```python
from build123d import *

# Parameters (mm, degrees)
EXTRUDE_1_DEPTH     = 20
SKETCH_2_R          = 1.1
CUT_EXTRUDE_2_DEPTH = 27.248809497
CUT_EXTRUDE_3_REACH = 31.682
SKETCH_3_W          = 30
SKETCH_3_H          = 15.1
FILLET_1_R          = 3
SKETCH_6_W          = 30.918408881
SKETCH_6_H          = 20
SKETCH_6_W_2        = 27.918408881
SKETCH_6_H_2        = 17
EXTRUDE_2_DEPTH     = 2.5
FILLET_2_R          = 3.5


with BuildPart() as part:
    # 草图1 → 凸台-拉伸1 (new body)
    with BuildSketch(Plane(origin=(0, 0, 0), x_dir=(1, 0, 0), z_dir=(0, 1, 0))):
        Polygon((-15, -8), (15, -0.520159915), (15, 8), (-15, 8), align=None)
    extrude(amount=EXTRUDE_1_DEPTH)

    # 草图2 → 切除-拉伸2 (cut, through all)
    with BuildSketch(Plane(origin=(0, 20, 0), x_dir=(1, 0, 0), z_dir=(0, 1, 0))):
        with Locations(Location((-13, 2, 0), (0, 0, 270))):
            Circle(SKETCH_2_R)
        with Locations(Location((-8.332097868, 3.791839748, 0), (0, 0, 270))):
            Circle(SKETCH_2_R)
        with Locations(Location((-3.664195735, 5.583679495, 0), (0, 0, 270))):
            Circle(SKETCH_2_R)
    extrude(amount=-CUT_EXTRUDE_2_DEPTH, mode=Mode.SUBTRACT)

    # 切除-拉伸3: up to this plane
    cut_extrude_3_end = Plane(origin=(0.637110354, 0, 2.555310061), z_dir=(0.24192189559966876, 0, 0.9702957262759963))
    # 草图3 → 切除-拉伸3 (cut, up to the surface)
    with BuildSketch(Plane(origin=(0, 0, -8), x_dir=(-1, 0, 0), z_dir=(0, 0, -1)), mode=Mode.PRIVATE) as cut_extrude_3_sk1:
        with Locations((0, 10)):
            Rectangle(SKETCH_3_W, SKETCH_3_H)
    cut_extrude_3_tool1 = split(extrude(cut_extrude_3_sk1.sketch, amount=-CUT_EXTRUDE_3_REACH, mode=Mode.PRIVATE), bisect_by=cut_extrude_3_end, keep=Keep.BOTH, mode=Mode.PRIVATE)
    add(cut_extrude_3_tool1.solids().sort_by_distance((0, 10, -8))[0], mode=Mode.SUBTRACT)

    # 圆角1
    fillet_1_edges = [part.edges().sort_by_distance(p)[0] for p in [
        (-15, 1.225, -8),
        (-15, 18.775, -8),
    ]]
    fillet(fillet_1_edges, radius=FILLET_1_R)

    # 草图6 → 凸台-拉伸2 (add)
    with BuildSketch(Plane(origin=(0.999993198, 0, 4.010753651), x_dir=(0.9702957262759964, 0, -0.2419218955996687), z_dir=(0.2419218955996687, 0, 0.9702957262759964))):
        with Locations((-1.030606619, 10)):
            Rectangle(SKETCH_6_W, SKETCH_6_H)
        with Locations((-1.030606619, 10)):
            Rectangle(SKETCH_6_W_2, SKETCH_6_H_2, mode=Mode.SUBTRACT)
    extrude(amount=EXTRUDE_2_DEPTH)

    # 圆角2
    fillet_2_edges = [part.edges().sort_by_distance(p)[0] for p in [
        (15, 1.225, -8),
        (15, 18.775, -8),
    ]]
    fillet(fillet_2_edges, radius=FILLET_2_R)


solid = part.part
```
Work out the finished part from the listing and answer in its coordinate system (mm). A direction names the side the tool comes from. Round coordinates to 2 decimals unless told otherwise and drop trailing zeros. Write each loop counter-clockwise with the first axis right and the second up, starting at its lowest first coordinate (ties: lowest second). Pieces come first, ordered by that corner, then holes.
1) Consider probe 1 along Y at (x, z) = (-11, 9); probe 2 along Y at (x, z) = (-6, -2.75); probe 3 along X at (y, z) = (1.85, -2). Determine where each line is inside the solid, lowest interval first.
2) Which of the six approach directions +Z, -Z, +X, -X, +Y, -Y give full straight-line access (tool end or side, diameter ignored) to faces 4 (the face through (0, 17.55, -2)), 5 (the face through (-13.246, 9.881, 8.833)), 6 (the face through (-3.616, 18.792, -6.683)), 7 (the face through (0, 19, -8)), 8 (the face through (13.843, 9.881, 2.079))?
3) Determine the mould class of faces 1 (the face through (-8.753, 1.242, -2.776)), 2 (the face through (-14.7, 9.9, 9.2)), 3 (the face through (-1, 0, 0)) for opening direction Z: pulls with the +Z half, pulls with the -Z half, needs draft (parallel to the pull), parting line crosses it, or undercut.
4) A cutting plane is placed at C-C on y = 4.5. Determine the outline of the cut face in (x, z), and give its area (3 significant figures).
5) A cutting plane is placed at A-A on z = -2. Determine the outline of the cut face in (x, y), and give its area (3 significant figures).
6) Flat-ended cylindrical pins translate along their axes: P1, Ø1.8, axis at x = -3.66, z = -5.58, coming from the -Y side; P2, Ø12, axis at x = 4.5, y = 9, coming from the +Z side. Find the tip coordinate at first contact, or state that the pin passes through.
7) A cutting plane is placed at D-D on z = 1.25. Determine the outline of the cut face in (x, y).
8) A cutting plane is placed at B-B on x = -12.5. Determine the outline of the cut face in (y, z), and give its area (3 significant figures).
Entries:
1. probe 1: y = 0 to 1.5, 18.5 to 20
1. probe 2: y = 0 to 2.45, 17.55 to 20
1. probe 3: x = -15 to -14.1, -11.9 to 15
2. face 4: -Z, -X
2. face 5: +X
2. face 6: +Y, -Y
2. face 7: -Z, +X, -X, +Y, -Y
2. face 8: +Z
3. face 1: undercut
3. face 2: pulls with the +Z half
3. face 3: needs draft
4. outline: (-15, 6.45) - (15, -1.03) - (15, 0.52) - (15.6, 2.95) - (14.15, 3.31) - (13.54, 0.88) - (-13.54, 7.64) - (-12.94, 10.06) - (-14.4, 10.43) - (-15, 8) - close
4. area: 53.9 mm2
5. outline: (-15, 0) - (-14.1, 0) - (-14.1, 2.45) - (-15, 2.45) - close; (-15, 17.55) - (-14.1, 17.55) - (-14.1, 20) - (-15, 20) - close; (-11.9, 0) - (15, 0) - (15, 2.45) - (-11.9, 2.45) - close; (-11.9, 17.55) - (15, 17.55) - (15, 20) - (-11.9, 20) - close
5. area: 136 mm2
6. P1: passes through
6. P2: stops at z = 4.63
7. outline: (-15, 0) - (15.18, 0) - (15.18, 20) - (-15, 20) - (-15, 17.55) - (5.87, 17.55) - (5.87, 2.45) - (-15, 2.45) - close; hole (12.07, 1.5) - (13.64, 1.5) - (13.64, 18.5) - (12.07, 18.5) - close
8. outline: (0, -7.96) - (2.45, -7.96) - (2.45, -2.98) - (0, -2.98) - close; (0, -1.02) - (2.45, -1.02) - (2.45, 5.83) - (17.55, 5.83) - (17.55, -1.02) - (20, -1.02) - (20, 9.95) - (18.5, 9.95) - (18.5, 7.38) - (1.5, 7.38) - (1.5, 9.95) - (0, 9.95) - close; (17.55, -7.96) - (20, -7.96) - (20, -2.98) - (17.55, -2.98) - close
8. area: 96.6 mm2
